Could you check a few things on this model? Use its own coordinates, in mm. A direction names the side the tool comes from. Give positions to 0.01 mm unless a question says otherwise; leave off trailing zeros. Order: outer loops, then holes, each group sorted by start corner. A loop starts at its lowest first (then second) coordinate and runs counter-clockwise, first axis right, second up. Notation, with made-up numbers: M 46.25,79 L 76.25,79 A16 cw 76.25,105 Z; hole C 6.25,4.5 d3. An arc over 180 degrees is marked long. Use a Markdown table: item, result. Add a question column.
Item 1: Suppose I cut it at D-D on z = -14. Write out the boundary of the cut face in (x, y).
Item 2: Suppose I cut it at C-C on y = 8. Write out the boundary of the cut face in (x, z).
Item 3: If we mould it in two halves opening along X, with no side actions, what happens to faces 3 (the face through (19.479, 18.966, -0.493)), 4 (the face through (-8, 25.5, -11)), 5 (the face through (20, 25, -11))? For each: released by +X, released by -X, zero draft, split by the parting line, or undercut.
Item 4: I'm going to push flat-ended pins straight in: pin 1 Ø13 at (x, y) = (0, 0) entering from +Z; pin 2 Ø3 at (y, z) = (24, -11) entering from +X; pin 3 Ø0.5 at (x, z) = (-27, -0.5) entering from -Y; pin 4 Ø4 at (x, z) = (8.5, -13) entering from -Y. Where does each tip first touch, or does it pass through?
Item 5: Suppose I cut it at B-B on x = 0. Write out the boundary of the cut face in (y, z).
Item 6: Suppose I cut it at A-A on y = 15. Write out the boundary of the cut face in (x, z), plus the area to 3 significant figures.
Item 7: For faces 1 (the face through (-0.867, -3.905, -21.507)), 2 (the face through (-8, 24.5, -11)), which set-ups out of +Z, -Z, +X, -X, +Y, -Y let a thin tool reach every point of the face, with its end or its side?
Item 8: If I drill on L1, parallel to Z at x = 10, y = 20; L2, parallel to Y at x = 15.5, z = -12.5; L3, parallel to Y at x = 0, z = -21.25, over which ranges is the centre line in solid material (lowest first)? Write a range as from..to.
from build123d import *

# Parameters (mm, degrees)
SKETCH_1_R                       = 4
SM_BASE_FLANGE_2_DEPTH           = 1
SM_EDGE_FLANGE_2_STRIP_W         = 5.4732
SM_EDGE_FLANGE_2_STRIP_H         = 1
SM_EDGE_FLANGE_2_STRIP_CUT_DEPTH = 55
SM_EDGE_FLANGE_2_DEPTH           = 55


# Sheet-metal steps are written as plain solids
with BuildPart() as part:
    # Sketch 1 → Базовая кромка2 (new body)
    with BuildSketch(Plane.XY):
        with BuildLine():
            Line((-20, 13), (-6.356958393, -4.856859066))
            ThreePointArc((-6.356958393, -4.856859066), (-1.096061515, -7.924559871), (4.8, -6.4))
            Line((4.8, -6.4), (24.8, 8.6))
            ThreePointArc((24.8, 8.6), (27.589466384, 17.529822128), (20, 23))
            Line((20, 23), (20, 25.5))
            Line((20, 25.5), (-20, 25.5))
            Line((-20, 25.5), (-35, 25.5))
            Line((-35, 25.5), (-35, 13))
            Line((-35, 13), (-20, 13))
        make_face()
        Circle(SKETCH_1_R, mode=Mode.SUBTRACT)
        with Locations((20, 15)):
            Circle(SKETCH_1_R, mode=Mode.SUBTRACT)
    extrude(amount=-SM_BASE_FLANGE_2_DEPTH)

    # Ребро-кромка2 strip (across the edge) → Ребро-кромка2 strip cut (cut)
    with BuildSketch(Plane(origin=(-35, 25.5, -1), x_dir=(0, -1, 0), z_dir=(1, 0, 0))):
        with Locations((-1, -0.5)):
            Rectangle(SM_EDGE_FLANGE_2_STRIP_W, SM_EDGE_FLANGE_2_STRIP_H)
    extrude(amount=SM_EDGE_FLANGE_2_STRIP_CUT_DEPTH, mode=Mode.SUBTRACT)

    # Ребро-кромка2 section (across the edge) → Ребро-кромка2 (add)
    with BuildSketch(Plane(origin=(-35, 25.5, -1), x_dir=(0, -1, 0), z_dir=(1, 0, 0))):
        with BuildLine():
            Line((0, 0.7366), (0, 10))
            Line((0, 10), (1, 10))
            Line((1, 10), (1, 0.7366))
            ThreePointArc((1, 0.7366), (1.215745145, 0.215745145), (1.7366, 0))
            Line((1.7366, 0), (1.7366, -1))
            ThreePointArc((1.7366, -1), (0.508638364, -0.491361636), (0, 0.7366))
        make_face()
    extrude(amount=SM_EDGE_FLANGE_2_DEPTH)

    # Зеркальное отражение1: part across face


with BuildPart() as part_1:
    add(part.part)
    add(part.part.mirror(Plane(origin=(-7.5, 25, -11), x_dir=(1, 0, 0), z_dir=(0, 0, -1))))


solid = part_1.part
Findings below:
| question | item | result |
|---|---|---|
| 1 | outline | M -35,24.5 L 20,24.5 L 20,25.5 L -35,25.5 Z |
| 2 | outline | M -16.18,-22 L 24,-22 L 24,-21 L -16.18,-21 Z; M -16.18,-1 L 24,-1 L 24,0 L -16.18,0 Z |
| 3 | face 3 | undercut |
| 3 | face 4 | zero draft |
| 3 | face 5 | released by +X |
| 4 | pin 1 | stops at z = 0 |
| 4 | pin 2 | stops at x = 20 |
| 4 | pin 3 | stops at y = 13 |
| 4 | pin 4 | stops at y = 24.5 |
| 5 | outline | M -8,-22 L -4,-22 L -4,-21 L -8,-21 Z; M -8,-1 L -4,-1 L -4,0 L -8,0 Z; M 4,-22 L 23.76,-22 A1.74 ccw 25.5,-20.26 L 25.5,-1.74 A1.74 ccw 23.76,0 L 4,0 L 4,-1 L 23.76,-1 A0.74 cw 24.5,-1.74 L 24.5,-20.26 A0.74 cw 23.76,-21 L 4,-21 Z |
| 6 | outline | M -35,-22 L 16,-22 L 16,-21 L -35,-21 Z; M -35,-1 L 16,-1 L 16,0 L -35,0 Z; M 24,-22 L 28,-22 L 28,-21 L 24,-21 Z; M 24,-1 L 28,-1 L 28,0 L 24,0 Z |
| 6 | area | 110 mm^2 |
| 7 | face 1 | +Z, -Z |
| 7 | face 2 | +X, -X, -Y |
| 8 | L1 | z = -22..-21, -1..0 |
| 8 | L2 | y = 24.5..25.5 |
| 8 | L3 | y = -8..-4, 4..25.19 |
